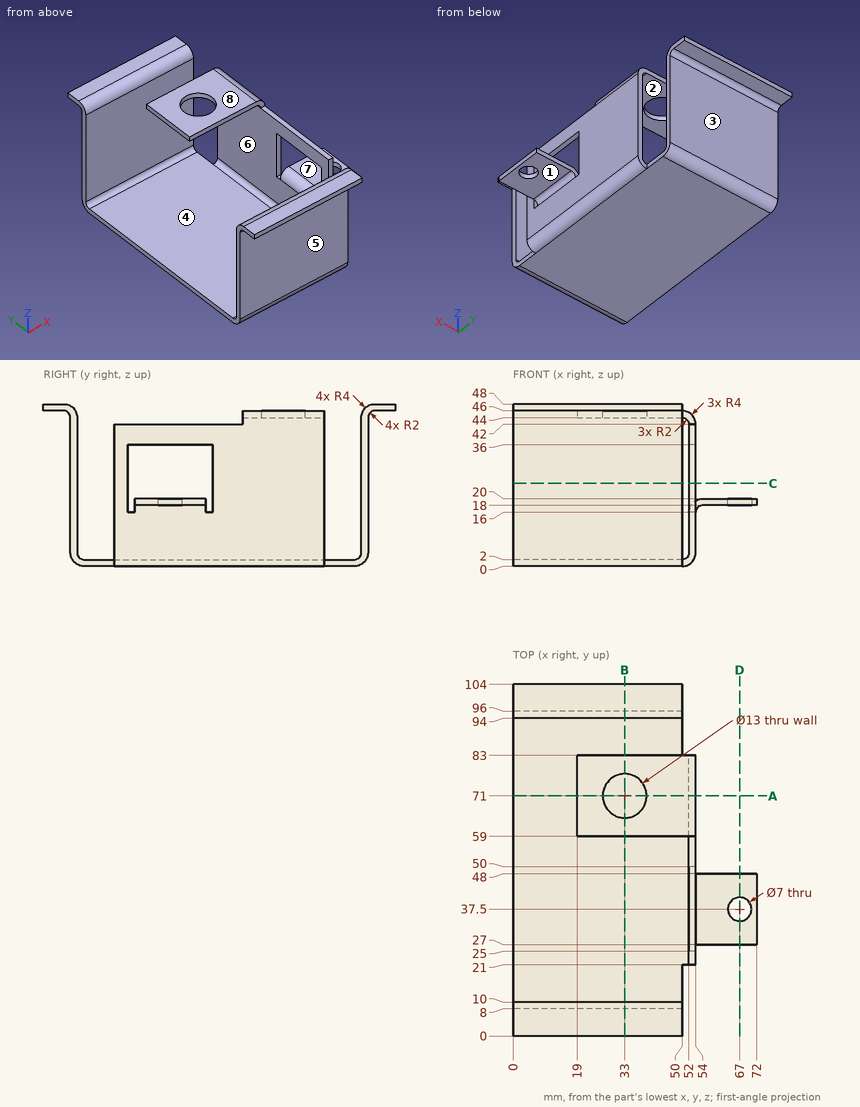
Design review of the part shown in the three views and the two pictorial views. Dimensions are in mm from the part's minimum x, y and z. A direction names the side the tool comes from. Round coordinates to 2 decimals unless told otherwise and drop trailing zeros. Write each loop counter-clockwise with the first axis right and the second up, starting at its lowest first coordinate (ties: lowest second). Pieces come first, ordered by that corner, then holes. Notation, with made-up numbers: (74, 20) -> (85, 20) arc R24 ccw to (85, 47) -> close; hole circle Ø5 at (64.25, 21.25). An arc over 180 degrees is marked (long way). Answer as a JSON object with one key per item and string values.
1. We need section D-D on x = 67. State the section outline as (y, z) points.
Results found:
{"outline": "(27, 18) -> (34, 18) -> (34, 20) -> (27, 20) -> close; (41, 18) -> (48, 18) -> (48, 20) -> (41, 20) -> close"}
2. We need section C-C on z = 24.5. State the section outline as (x, y) points.
Results found:
{"outline": "(0, 8) -> (50, 8) -> (50, 10) -> (0, 10) -> close; (0, 94) -> (50, 94) -> (50, 96) -> (0, 96) -> close; (52, 21) -> (54, 21) -> (54, 25) -> (52, 25) -> close; (52, 50) -> (54, 50) -> (54, 83) -> (52, 83) -> close"}
3. We need section B-B on x = 33. State the section outline as (y, z) points, and give its area (3 significant figures).
Results found:
{"outline": "(0, 46) -> (6, 46) arc R2 cw to (8, 44) -> (8, 4) arc R4 ccw to (12, 0) -> (92, 0) arc R4 ccw to (96, 4) -> (96, 44) arc R2 cw to (98, 46) -> (104, 46) -> (104, 48) -> (98, 48) arc R4 ccw to (94, 44) -> (94, 4) arc R2 cw to (92, 2) -> (12, 2) arc R2 cw to (10, 4) -> (10, 44) arc R4 ccw to (6, 48) -> (0, 48) -> close; (59, 44) -> (64.5, 44) -> (64.5, 46) -> (59, 46) -> close; (77.5, 44) -> (83, 44) -> (83, 46) -> (77.5, 46) -> close", "area": "404 mm^2"}
4. The part is to be moulded in two halves that separate along Y. For the marked faces 1, 2 and 3, say which applies: pulls with the +Y half, pulls with the -Y half, needs draft (parallel to the pull), parting line crosses it, or undercut.
Results found:
{"face 1": "needs draft", "face 2": "undercut", "face 3": "pulls with the +Y half"}
5. We need section A-A on y = 71. State the section outline as (x, z) points.
Results found:
{"outline": "(0, 0) -> (50, 0) arc R4 ccw to (54, 4) -> (54, 42) arc R4 ccw to (50, 46) -> (39.5, 46) -> (39.5, 44) -> (50, 44) arc R2 cw to (52, 42) -> (52, 4) arc R2 cw to (50, 2) -> (0, 2) -> close; (19, 44) -> (26.5, 44) -> (26.5, 46) -> (19, 46) -> close"}
6. Machinability: for the marked faces 4, 5, 6, 7 and 8, which of the approach directions +Z, -Z, +X, -X, +Y, -Y give a long, thin tool a straight path to every point of the face, cutting with its end or side? Answer none if there is none.
Results found:
{"face 4": "-X", "face 5": "-Z, +X, -X, -Y", "face 6": "-X, +Y, -Y", "face 7": "+Z, +X, -X, +Y, -Y", "face 8": "+Z, +X, -X"}
7. To check wall thickness, follow line 1 along Y through (x, z) = (38.5, 28); line 2 along Y through (x, z) = (67, 19); line 3 along Y through (x, z) = (33, 44.95). State the ranges of each line that lie inside material, in increasing order.
Results found:
{"line 1": "y = 8 to 10, 94 to 96", "line 2": "y = 27 to 34, 41 to 48", "line 3": "y = 7.76 to 9.89, 59 to 64.5, 77.5 to 83, 94.11 to 96.24"}
8. Clearance check with flat-ended pins moving along their axes: pin 1 (15 mm diameter, centred on x = 24, y = 67.5, fed in from +Z); pin 2 (1.6 mm diameter, centred on x = 53.5, y = 37, fed in from -Z); pin 3 (1.8 mm diameter, centred on x = 19, y = 101.5, fed in from -Z). State where each tip first meets the part, or that it passes through.
Results found:
{"pin 1": "stops at z = 46", "pin 2": "stops at z = 1.05", "pin 3": "stops at z = 46"}
